Drawing for the job (mm, zero at the part's lowest x, y, z). A direction names the side the tool comes from. Coordinates: 2 decimals unless noted, no trailing zeros. Loops run counter-clockwise (first coordinate to the right, second up) from the corner with the lowest first, then second, coordinate; pieces in that order, holes last. Notation, with made-up numbers: (-2.75, 32) -> (11.25, 32) arc R29 cw to (11.25, 56) -> close; hole circle Ø6 at (-0.75, 39). An arc over 180 degrees is marked (long way). Write item = value, one per line. Start each with the question number.
(1) Flat gauge pins, fed straight in: P1, Ø0.5, axis at y = 1.5, z = 6, coming from the +X side; P2, Ø2.5, axis at x = 2, z = 4.5, coming from the -Y side; P3, Ø1, axis at x = 1.5, z = 5, coming from the +Y side; P4, Ø1.1, axis at x = 4, y = 3.5, coming from the +Z side. Where does each tip first touch, or does it go through?
(2) Band-saw the part on A-A (y = 3.75). Write the cut outline in (x, z), and give its area (3 significant figures).
(3) Band-saw the part on B-B (z = 1.5). Write the cut outline in (x, y).
(4) Drill centre lines: line 1 (X direction, y = 0.65, z = 1.5); line 2 (Y direction, x = 2.15, z = 5.5); line 3 (X direction, y = 2.3, z = 7.25). Where is each one in solid material? Low to high. Write a range as from..to.
(5) Band-saw the part on C-C (x = 1.4). Write the cut outline in (y, z), and give its area (3 significant figures).
(6) Tool access for the marked faces 1, 2, 3, 4 and 5: list every direction of +Z, -Z, +X, -X, +Y, -Y with a clear straight run to the whole face (end or side of a thin tool).
(7) Band-saw the part on D-D (y = 1.2). Write the cut outline in (x, z).
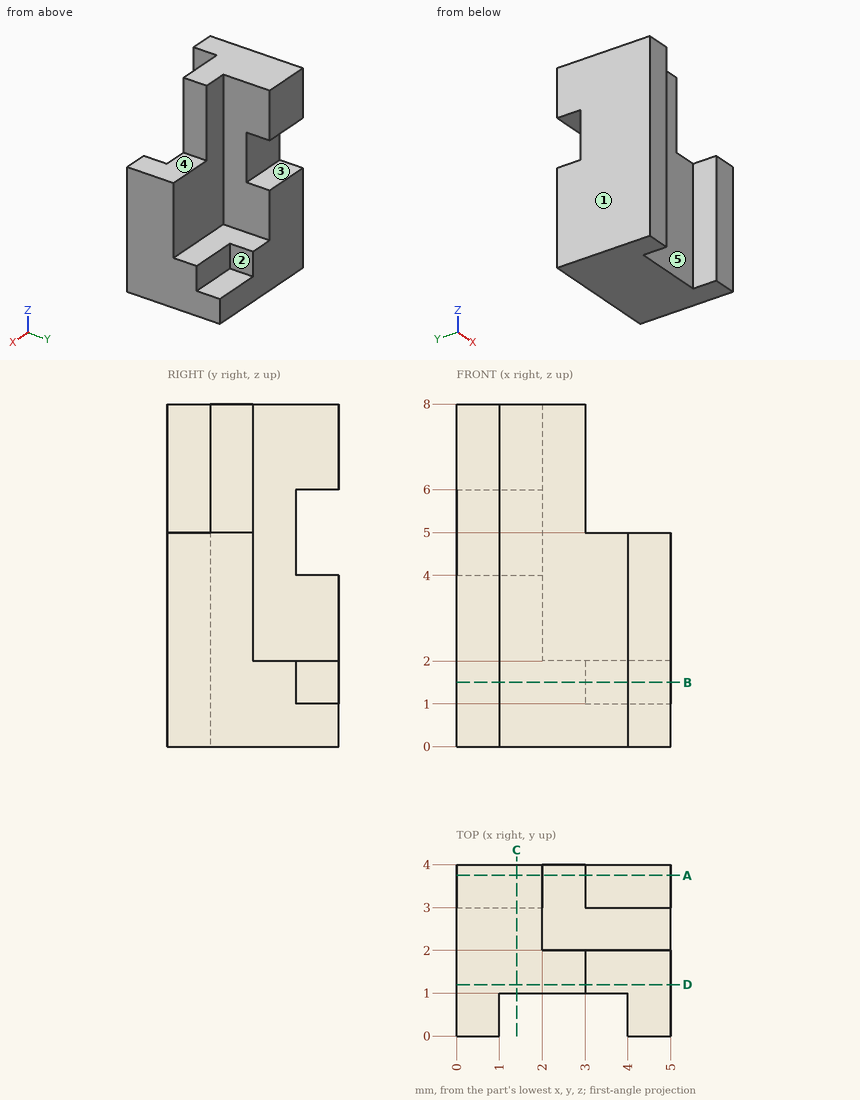
Findings below:
q1.P1 = 3
q1.P2 = 0
q1.P3 = 3
q1.P4 = 2
q2.outline = (0, 0) -> (5, 0) -> (5, 1) -> (3, 1) -> (3, 2) -> (2, 2) -> (2, 4) -> (0, 4) -> close; (0, 6) -> (2, 6) -> (2, 8) -> (0, 8) -> close
q2.area = 16.0 mm²
q3.outline = (0, 0) -> (1, 0) -> (1, 1) -> (4, 1) -> (4, 0) -> (5, 0) -> (5, 3) -> (3, 3) -> (3, 4) -> (0, 4) -> close
q4.line_1 = 0..1, 4..5
q4.line_2 = 1..2
q4.line_3 = 0..2
q5.outline = (1, 0) -> (4, 0) -> (4, 4) -> (3, 4) -> (3, 6) -> (4, 6) -> (4, 8) -> (1, 8) -> close
q5.area = 22.0 mm²
q6.face_1 = +Z, -Z, -X, +Y, -Y
q6.face_2 = +Z, +X, +Y
q6.face_3 = +X, -X, +Y
q6.face_4 = +Z, +X, +Y, -Y
q6.face_5 = +Z, -Z, -Y
q7.outline = (0, 0) -> (5, 0) -> (5, 5) -> (3, 5) -> (3, 8) -> (0, 8) -> close
